Read the model definition and answer for the solid it produces. Units are mm, in the model's axes. A direction names the side the tool comes from. Coordinates: 2 decimals unless noted, no trailing zeros. Loops run counter-clockwise (first coordinate to the right, second up) from the corner with the lowest first, then second, coordinate; pieces in that order, holes last. Notation, with made-up numbers: (82, 35) - (136, 35) arc R13 cw to (136, 51) - close; hole circle Ø3 at (-1.5, -23.75). An arc over 180 degrees is marked (long way). Use one line per item in the form item = value. Start each with the question number.
1) A cutting plane is placed at D-D (y = 22.5). Give the vertices of the cut face in (x, z).
2) A cutting plane is placed at A-A (x = -4.5). Give the vertices of the cut face in (y, z).
3) The mould has two halves that part along Y. Classify faces 1 (the face through (-32, 7.5, 8)), 2 (the face through (-29, 0, 7)), 3 (the face through (-27, 4, 9)): released by +Y, released by -Y, zero draft, split by the parting line, or undercut.
4) A cutting plane is placed at C-C (x = -25). Give the vertices of the cut face in (y, z), and give its area (3 significant figures).
5) Each of these flat-tipped pins is pushed along its axis until it touches: P1, Ø5, axis at x = -23.5, z = 9.5, coming from the -Y side; P2, Ø1.6, axis at y = 9, z = 9, coming from the -X side; P3, Ø4, axis at x = -44.5, z = 7.5, coming from the -Y side; P4, Ø3, axis at y = 15, z = 3, coming from the -X side. Where does it stop, or does it pass through?
6) Consider line 1 (X direction, y = 25.25, z = 7.5); line 2 (Y direction, x = -32.5, z = 10.75); line 3 (Y direction, x = -13, z = 7.5). Determine where each line is inside the solid, lowest interval first.
7) A cutting plane is placed at B-B (z = 4.25). State how many separate pieces and enclosed holes the cut face has, and give its area (3 significant figures).
8) Which of the six approach directions +Z, -Z, +X, -X, +Y, -Y give full straight-line access (tool end or side, diameter ignored) to faces 4 (the face through (-40, 9.5, 8)), 5 (the face through (-4, 22, 5)), 6 (the face through (-46, 22, 5)), 7 (the face through (-27.2, 8, 9))?
from build123d import *

# Parameters (mm, degrees)
SKETCH1_W            = 50
SKETCH1_H            = 26
BOSS_EXTRUDE1_DEPTH  = 16
SKETCH2_W            = 8.5
SKETCH2_H            = 22
CUT_EXTRUDE1_DEPTH   = 59.583274064
SKETCH3_W            = 8.5
SKETCH3_H            = 22
CUT_EXTRUDE2_DEPTH   = 59.583274064
SKETCH4_W            = 12
SKETCH4_H            = 10.5
CUT_EXTRUDE3_DEPTH   = 52.217672731
SKETCH5_W            = 14.5
SKETCH5_H            = 7.5
BOSS_EXTRUDE2_DEPTH  = 12
SKETCH6_W            = 1.3
SKETCH6_H            = 2
BOSS_EXTRUDE3_DEPTH  = 12
SKETCH7_W            = 1.3
SKETCH7_H            = 2
BOSS_EXTRUDE4_DEPTH  = 12
SKETCH8_W            = 1.3
SKETCH8_H            = 2
BOSS_EXTRUDE5_DEPTH  = 12
SKETCH9_W            = 1.3
SKETCH9_H            = 2
BOSS_EXTRUDE6_DEPTH  = 12
SKETCH10_W           = 1.3
SKETCH10_H           = 2
BOSS_EXTRUDE7_DEPTH  = 12
SKETCH11_W           = 14.5
SKETCH11_H           = 7.5
BOSS_EXTRUDE8_DEPTH  = 12
SKETCH12_W           = 1.3
SKETCH12_H           = 2
BOSS_EXTRUDE9_DEPTH  = 12
SKETCH13_W           = 1.3
SKETCH13_H           = 2
BOSS_EXTRUDE10_DEPTH = 12
SKETCH14_W           = 1.3
SKETCH14_H           = 2
BOSS_EXTRUDE11_DEPTH = 12
SKETCH15_W           = 1.3
SKETCH15_H           = 2
BOSS_EXTRUDE12_DEPTH = 12
SKETCH16_W           = 1.3
SKETCH16_H           = 2
BOSS_EXTRUDE13_DEPTH = 12
SKETCH17_R           = 1.7
CUT_EXTRUDE4_DEPTH   = 59.318093247
SKETCH18_R           = 1.7
CUT_EXTRUDE5_DEPTH   = 59.318093247
CHAMFER2_SIZE        = 2


with BuildPart() as part:
    # Sketch1 → Boss-Extrude1 (new body)
    with BuildSketch(Plane(origin=(0, 0, -1), x_dir=(-1, 0, 0), z_dir=(0, 0, -1))):
        with Locations((25, 13)):
            Rectangle(SKETCH1_W, SKETCH1_H)
    extrude(amount=-BOSS_EXTRUDE1_DEPTH)

    # Sketch2 → Cut-Extrude1 (cut, through all)
    with BuildSketch(Plane(origin=(0, 0, -1), x_dir=(-1, 0, 0), z_dir=(0, 0, -1))):
        with Locations((45.75, 11)):
            Rectangle(SKETCH2_W, SKETCH2_H)
    extrude(amount=-CUT_EXTRUDE1_DEPTH, mode=Mode.SUBTRACT)

    # Sketch3 → Cut-Extrude2 (cut, through all)
    with BuildSketch(Plane(origin=(0, 0, -1), x_dir=(-1, 0, 0), z_dir=(0, 0, -1))):
        with Locations((4.25, 11)):
            Rectangle(SKETCH3_W, SKETCH3_H)
    extrude(amount=-CUT_EXTRUDE2_DEPTH, mode=Mode.SUBTRACT)

    # Sketch4 → Cut-Extrude3 (cut, through all)
    with BuildSketch(Plane.ZY.offset(41.5)):
        with Locations((9, 5.25)):
            Rectangle(SKETCH4_W, SKETCH4_H)
    extrude(amount=-CUT_EXTRUDE3_DEPTH, mode=Mode.SUBTRACT)

    # Sketch5 → Boss-Extrude2 (add)
    with BuildSketch(Plane.XY.offset(3)):
        with Locations((-15.75, 3.75)):
            Rectangle(SKETCH5_W, SKETCH5_H)
    extrude(amount=BOSS_EXTRUDE2_DEPTH)

    # Sketch6 → Boss-Extrude3 (add)
    with BuildSketch(Plane.XY.offset(3)):
        with Locations((-9.85, 8.5)):
            Rectangle(SKETCH6_W, SKETCH6_H)
    extrude(amount=BOSS_EXTRUDE3_DEPTH)

    # Sketch7 → Boss-Extrude4 (add)
    with BuildSketch(Plane.XY.offset(3)):
        with Locations((-12.85, 8.5)):
            Rectangle(SKETCH7_W, SKETCH7_H)
    extrude(amount=BOSS_EXTRUDE4_DEPTH)

    # Sketch8 → Boss-Extrude5 (add)
    with BuildSketch(Plane.XY.offset(3)):
        with Locations((-15.85, 8.5)):
            Rectangle(SKETCH8_W, SKETCH8_H)
    extrude(amount=BOSS_EXTRUDE5_DEPTH)

    # Sketch9 → Boss-Extrude6 (add)
    with BuildSketch(Plane.XY.offset(3)):
        with Locations((-18.85, 8.5)):
            Rectangle(SKETCH9_W, SKETCH9_H)
    extrude(amount=BOSS_EXTRUDE6_DEPTH)

    # Sketch10 → Boss-Extrude7 (add)
    with BuildSketch(Plane.XY.offset(3)):
        with Locations((-21.85, 8.5)):
            Rectangle(SKETCH10_W, SKETCH10_H)
    extrude(amount=BOSS_EXTRUDE7_DEPTH)

    # Sketch11 → Boss-Extrude8 (add)
    with BuildSketch(Plane.XY.offset(3)):
        with Locations((-34.25, 3.75)):
            Rectangle(SKETCH11_W, SKETCH11_H)
    extrude(amount=BOSS_EXTRUDE8_DEPTH)

    # Sketch12 → Boss-Extrude9 (add)
    with BuildSketch(Plane.XY.offset(3)):
        with Locations((-27.85, 8.5)):
            Rectangle(SKETCH12_W, SKETCH12_H)
    extrude(amount=BOSS_EXTRUDE9_DEPTH)

    # Sketch13 → Boss-Extrude10 (add)
    with BuildSketch(Plane.XY.offset(3)):
        with Locations((-30.85, 8.5)):
            Rectangle(SKETCH13_W, SKETCH13_H)
    extrude(amount=BOSS_EXTRUDE10_DEPTH)

    # Sketch14 → Boss-Extrude11 (add)
    with BuildSketch(Plane.XY.offset(3)):
        with Locations((-33.85, 8.5)):
            Rectangle(SKETCH14_W, SKETCH14_H)
    extrude(amount=BOSS_EXTRUDE11_DEPTH)

    # Sketch15 → Boss-Extrude12 (add)
    with BuildSketch(Plane.XY.offset(3)):
        with Locations((-36.85, 8.5)):
            Rectangle(SKETCH15_W, SKETCH15_H)
    extrude(amount=BOSS_EXTRUDE12_DEPTH)

    # Sketch16 → Boss-Extrude13 (add)
    with BuildSketch(Plane.XY.offset(3)):
        with Locations((-39.85, 8.5)):
            Rectangle(SKETCH16_W, SKETCH16_H)
    extrude(amount=BOSS_EXTRUDE13_DEPTH)

    # Sketch17 → Cut-Extrude4 (cut, through all)
    with BuildSketch(Plane(origin=(0, 26, 0), x_dir=(-1, 0, 0), z_dir=(0, 1, 0))):
        with Locations(Location((4.5, 7.5, 0), (0, 0, 90))):
            Circle(SKETCH17_R)
    extrude(amount=-CUT_EXTRUDE4_DEPTH, mode=Mode.SUBTRACT)

    # Sketch18 → Cut-Extrude5 (cut, through all)
    with BuildSketch(Plane(origin=(0, 26, 0), x_dir=(-1, 0, 0), z_dir=(0, 1, 0))):
        with Locations(Location((45.449445698, 7.5, 0), (0, 0, 90))):
            Circle(SKETCH18_R)
    extrude(amount=-CUT_EXTRUDE5_DEPTH, mode=Mode.SUBTRACT)

    # Chamfer2
    chamfer2_edges = [part.edges().sort_by_distance(p)[0] for p in [
        (-39.85, 9.5, 15),
        (-38.35, 7.5, 15),
        (-36.85, 9.5, 15),
        (-35.35, 7.5, 15),
        (-33.85, 9.5, 15),
        (-32.35, 7.5, 15),
        (-30.85, 9.5, 15),
        (-29.35, 7.5, 15),
        (-27.85, 9.5, 15),
        (-27.1, 7.5, 15),
        (-41, 7.5, 15),
        (-25, 10.5, 15),
    ]]
    chamfer(chamfer2_edges, length=CHAMFER2_SIZE - 0.0001)  # a hair under: the kernel refuses the full size


solid = part.part
Found:
q1.outline = (-50, -1) - (0, -1) - (0, 15) - (-50, 15) - close; hole circle Ø3.4 at (-45.45, 7.5); hole circle Ø3.4 at (-4.5, 7.5)
q2.outline = (22, -1) - (26, -1) - (26, 5.8) - (22, 5.8) - close; (22, 9.2) - (26, 9.2) - (26, 15) - (22, 15) - close
q3.face_1 = undercut
q3.face_2 = released by -Y
q3.face_3 = zero draft
q4.outline = (0, -1) - (26, -1) - (26, 15) - (12.5, 15) - (10.5, 13) - (10.5, 3) - (0, 3) - close
q4.area = 288 mm^2
q5.P1 = 0
q5.P2 = -40.5
q5.P3 = 22
q5.P4 = -41.5
q6.line_1 = -50 to -47.15, -43.75 to -6.2, -2.8 to 0
q6.line_2 = 0 to 7.5, 10.5 to 26
q6.line_3 = 0 to 9.5, 10.5 to 26
q7.separate_pieces = 3
q7.enclosed_holes = 0
q7.area = 823 mm^2
q8.face_4 = +Z, +X, -X
q8.face_5 = +Z, -Z, +X, -Y
q8.face_6 = +Z, -Z, -X, -Y
q8.face_7 = +Z
